Solid Edge part; units mm, degrees
sketch "Sketch1" plane through (0, 0, 0) normal (0, -1, 0) x (1, 0, 0)
  line L0 (-28.5, 0) -> (28.5, 0)
  line L1 (28.5, 0) -> (28.5, 9)
  line L2 (28.5, 9) -> (48.5, 9)
  line L3 (48.5, 9) -> (48.5, 7)
  line L4 (48.5, 7) -> (30.5, 7)
  line L5 (30.5, 7) -> (30.5, -2)
  line L6 (30.5, -2) -> (-30.5, -2)
  line L7 (-30.5, -2) -> (-30.5, 0)
  line L8 (-28.5, 0) -> (-30.5, 0)
extrude "Protrusion1" add sketch "Sketch1" against normal blind 86
sketch "Sketch2" plane through (0, 43, -2) normal (0, 0, -1) x (0, -1, 0)
  line L0 (-43, 30.5) -> (-43, -30.5)
  line L1 (-43, -30.5) -> (-45, -30.5)
  line L2 (-45, -30.5) -> (-45, 30.5)
  line L3 (-45, 30.5) -> (-43, 30.5)
  line L4 (45, -30.5) -> (45, 30.5)
  line L5 (45, 30.5) -> (43, 30.5)
  line L6 (43, 30.5) -> (43, -30.5)
  line L7 (43, -30.5) -> (45, -30.5)
extrude "ExtrudedProtrusion_2" add sketch "Sketch2" against normal blind 11
sketch "Sketch3" plane through (0, -2, 3.5) normal (0, -1, 0) x (1, 0, 0)
  line L0 (28.5, 3.5) -> (-30.5, 3.5)
  line L1 (-30.5, 3.5) -> (-30.5, 5.5)
  line L2 (-30.5, 5.5) -> (28.5, 5.5)
  line L3 (28.5, 5.5) -> (28.5, 3.5)
extrude "ExtrudedProtrusion_3" add sketch "Sketch3" along normal blind 20
sketch "Sketch4" plane through (0, 88, 3.5) normal (0, 1, 0) x (-1, 0, 0)
  line L0 (-28.5, 3.5) -> (30.5, 3.5)
  line L1 (30.5, 3.5) -> (30.5, 5.5)
  line L2 (30.5, 5.5) -> (-28.5, 5.5)
  line L3 (-28.5, 5.5) -> (-28.5, 3.5)
extrude "ExtrudedProtrusion_4" add sketch "Sketch4" along normal blind 20
sketch "Sketch5" plane through (9, 43, 9) normal (0, 0, 1) x (1, 0, 0)
  line L0 (19.5, -55) -> (-39.5, -55)
  line L1 (-39.5, -55) -> (-39.5, -65)
  line L2 (-39.5, -65) -> (19.5, -65)
  line L3 (19.5, -65) -> (19.5, -55)
  line L4 (19.5, 55) -> (-39.5, 55)
  line L5 (-39.5, 55) -> (-39.5, 65)
  line L6 (-39.5, 65) -> (19.5, 65)
  line L7 (19.5, 65) -> (19.5, 55)
extrude "Cutout1" cut sketch "Sketch5" against normal up to next
Part model, mm, in its own coordinate system. A direction names the side the tool comes from. Coordinates: 2 decimals unless noted, no trailing zeros. Loops run counter-clockwise (first coordinate to the right, second up) from the corner with the lowest first, then second, coordinate; pieces in that order, holes last. Notation, with made-up numbers: (42, -36) - (99, -36) arc R19 ccw to (99, -5) - close; hole circle Ø5 at (17, 0). An arc over 180 degrees is marked (long way). Write each question's results on one line, items separated by ' | '. Start each with the question number.
Q1. Slice it at A-A on y = 60.5. Give the cut face in (x, z).
Q2. Drop flat-ended pins along their axis: pin 1 Ø3.5 at (y, z) = (36, 3) entering from +X; pin 2 Ø0.6 at (y, z) = (93.5, 8.5) entering from +X; pin 3 Ø8 at (x, y) = (0, 95) entering from -Z. Give the stop position or say it passes through.
Q3. Slice it at C-C on x = -7. Give the cut face in (y, z).
Q4. Two-plate mould, pull along Y, no slides. Class faces 1 (the flat face through (-1, 86, 4)), 2 (the flat face through (-1, -7, 7)): +Y half, -Y half, draft (parallel to the pull), parting line (faces both ways), or undercut.
Q5. Probe line 1 along Y through (x, z) = (-23, 4.5); line 2 along Y through (x, z) = (5.5, 7.5); line 3 along Z through (x, y) = (26, 72.5). List the from-to ranges inside material, lowest first.
Q6. Which spindle directions (+Z, -Z, +X, -X, +Y, -Y) get a long thin tool onto all of the face, cutting with end or side? Do faces 3 (the flat face through (-1, 42, 0)), 4 (the flat face through (-1, 93, 7)), 5 (the flat face through (40, 42, 7)). Say none if no direction does.
Q7. Slice it at D-D on x = 36. Give the cut face in (y, z).
Q8. Slice it at B-B on z = 2.25. Give the cut face in (x, y), and give its area (3 significant figures).
Answer:
1) outline: (-30.5, -2) - (30.5, -2) - (30.5, 7) - (48.5, 7) - (48.5, 9) - (28.5, 9) - (28.5, 0) - (-30.5, 0) - close
2) pin 1: stops at x = 30.5 | pin 2: stops at x = 28.5 | pin 3: stops at z = 7
3) outline: (-12, 7) - (-2, 7) - (-2, -2) - (88, -2) - (88, 7) - (98, 7) - (98, 9) - (86, 9) - (86, 0) - (0, 0) - (0, 9) - (-12, 9) - close
4) face 1: undercut | face 2: draft
5) line 1: y = -2 to 0, 86 to 88 | line 2: y = -12 to 0, 86 to 98 | line 3: z = -2 to 0
6) face 3: +Z, -X | face 4: -Z, +X, -X, +Y | face 5: -Z, +X, +Y, -Y
7) outline: (0, 7) - (86, 7) - (86, 9) - (0, 9) - close
8) outline: (-30.5, -2) - (30.5, -2) - (30.5, 88) - (-30.5, 88) - (-30.5, 86) - (28.5, 86) - (28.5, 0) - (-30.5, 0) - close | area: 416 mm2
